from build123d import *

# Parameters (mm, degrees)
ESQUISSE1_R        = 0.825
ESQUISSE1_R_2      = 0.75
ESQUISSE1_W        = 38.13
ESQUISSE1_H        = 18.5
ESQUISSE1_W_2      = 17
ESQUISSE1_H_2      = 9
ESQUISSE1_W_3      = 2
ESQUISSE1_H_3      = 5
BOSS_EXTRU_1_DEPTH = 2
CHANFREIN1_SIZE    = 2
ESQUISSE2_R        = 1.65
BOSS_EXTRU_2_DEPTH = 2
CONG_1_R           = 2
CONG_4_R           = 2


with BuildPart() as part:
    # Esquisse1 → Boss.-Extru.1 (new body)
    # profile 1 of 3: a face of its own
    with BuildSketch(Plane(origin=(0, 0, 0), x_dir=(1, 0, 0), z_dir=(0, 1, 0))):
        Polygon((-11.996169772, 14.323981369), (31.213830228, 14.323981369), (35.738830228, 9.823981369), (83.213830228, 9.823981369), (83.213830228, -3.176018631), (35.738830228, -3.176018631), (31.213830228, -7.676018631), (-11.996169772, -7.676018631), align=None)
        with Locations(Location((-10.726169772, 11.303981369, 0), (0, 0, 270))):
            Circle(ESQUISSE1_R, mode=Mode.SUBTRACT)
        with Locations(Location((29.943830228, 11.303981369, 0), (0, 0, 270))):
            Circle(ESQUISSE1_R, mode=Mode.SUBTRACT)
        with Locations(Location((29.943830228, -4.656018631, 0), (0, 0, 270))):
            Circle(ESQUISSE1_R, mode=Mode.SUBTRACT)
        with Locations(Location((-10.726169772, -4.656018631, 0), (0, 0, 270))):
            Circle(ESQUISSE1_R, mode=Mode.SUBTRACT)
        with Locations(Location((33.943830228, 3.323981369, 0), (0, 0, 270))):
            Circle(ESQUISSE1_R_2, mode=Mode.SUBTRACT)
        with Locations(Location((54.533830228, 3.323981369, 0), (0, 0, 270))):
            Circle(ESQUISSE1_R_2, mode=Mode.SUBTRACT)
        with Locations(Location((60.533830228, 3.323981369, 0), (0, 0, 270))):
            Circle(ESQUISSE1_R_2, mode=Mode.SUBTRACT)
        with Locations(Location((81.123830228, 3.323981369, 0), (0, 0, 270))):
            Circle(ESQUISSE1_R_2, mode=Mode.SUBTRACT)
        with Locations((9.608830228, 3.323981369)):
            Rectangle(ESQUISSE1_W, ESQUISSE1_H, mode=Mode.SUBTRACT)
        with Locations((44.238830228, 3.323981369)):
            Rectangle(ESQUISSE1_W_2, ESQUISSE1_H_2, mode=Mode.SUBTRACT)
        with Locations((70.828830228, 3.323981369)):
            Rectangle(ESQUISSE1_W_2, ESQUISSE1_H_2, mode=Mode.SUBTRACT)
    # profile 2 of 3: a face of its own
    with BuildSketch(Plane(origin=(0, 0, 0), x_dir=(1, 0, 0), z_dir=(0, 1, 0))):
        with Locations((-12.996169772, 3.323981369)):
            Rectangle(ESQUISSE1_W_3, ESQUISSE1_H_3)
    # profile 3 of 3: a face of its own
    with BuildSketch(Plane(origin=(0, 0, 0), x_dir=(1, 0, 0), z_dir=(0, 1, 0))):
        with Locations((84.213830228, 3.323981369)):
            Rectangle(ESQUISSE1_W_3, ESQUISSE1_H_3)
    extrude(amount=BOSS_EXTRU_1_DEPTH)

    # Chanfrein1
    chanfrein1_edges = [part.edges().sort_by_distance(p)[0] for p in [
        (83.213830228, 1, -9.823981369),
        (83.213830228, 1, 3.176018631),
    ]]
    chamfer(chanfrein1_edges, length=CHANFREIN1_SIZE)

    # Esquisse2 → Boss.-Extru.2 (add)
    with BuildSketch(Plane(origin=(85.213830228, 0, 0), x_dir=(0, 0, -1), z_dir=(1, 0, 0))):
        Polygon((5.823981369, 0), (0.823981369, 0), (2.323981369, -2), (2.323981369, -9), (0.823981369, -9), (0.823981369, -14), (5.823981369, -14), (5.823981369, -9), (4.323981369, -9), (4.323981369, -2), align=None)
        with Locations((3.323981369, -11.5)):
            Circle(ESQUISSE2_R, mode=Mode.SUBTRACT)
    boss_extru_2 = extrude(amount=-BOSS_EXTRU_2_DEPTH)

    # Symétrie1: Boss.-Extru.2 across plane
    add(boss_extru_2.mirror(Plane(origin=(35.738830228, 2, 0), x_dir=(0, 0, 1), z_dir=(-1, 0, 0))))

    # Congé1
    # the kernel refuses this fillet: 2 mm, written as the material it takes off along each edge
    with BuildSketch(Plane(origin=(90.213830228, -14, -5.823981369), x_dir=(0, 0, 1), z_dir=(-1, 0, 0)), Plane(origin=(90.213830228, -14, -0.823981369), x_dir=(0, 1, 0), z_dir=(-1, 0, 0))) as cong_1_piece_1:
        with BuildLine():
            CenterArc((CONG_1_R, CONG_1_R), CONG_1_R, 180, 90)
            Line((0, CONG_1_R), (-CONG_1_R * 0.02, CONG_1_R))
            Line((-CONG_1_R * 0.02, CONG_1_R), (-CONG_1_R * 0.02, -CONG_1_R * 0.02))
            Line((-CONG_1_R * 0.02, -CONG_1_R * 0.02), (CONG_1_R, -CONG_1_R * 0.02))
            Line((CONG_1_R, -CONG_1_R * 0.02), (CONG_1_R, 0))
        make_face()
    extrude(amount=12, mode=Mode.SUBTRACT)
    with BuildSketch(Plane(origin=(90.055059411, -9, -5.823981369), x_dir=(0, -1, 0), z_dir=(-1, 0, 0)), Plane(origin=(-18.577398955, -9, -0.823981369), x_dir=(0, -1, 0), z_dir=(1, 0, 0))) as cong_1_piece_2:
        with BuildLine():
            CenterArc((1.936491673, 2), CONG_1_R, 194.477512186, 75.522487814)
            Line((0, 1.5), (-0.038729833, 1.49))
            ThreePointArc((-0.038729833, 1.49), (-0.04, 0.75), (-0.04, 0))
            Line((-0.04, 0), (0, -0.04))
            Line((0, -0.04), (1.936491673, -0.04))
            Line((1.936491673, -0.04), (1.936491673, 0))
        make_face()
    extrude(amount=11.682458366, mode=Mode.SUBTRACT)
    with BuildSketch(Plane(origin=(90.055059411, -9, -0.823981369), x_dir=(0, -1, 0), z_dir=(-1, 0, 0)), Plane(origin=(-18.577398955, -9, -5.823981369), x_dir=(0, -1, 0), z_dir=(1, 0, 0))) as cong_1_piece_3:
        with BuildLine():
            CenterArc((1.936491673, -2), CONG_1_R, 90, 75.522487814)
            Line((0, -1.5), (-0.038729833, -1.49))
            ThreePointArc((-0.038729833, -1.49), (-0.04, -0.75), (-0.04, 0))
            Line((-0.04, 0), (0, 0.04))
            Line((0, 0.04), (1.936491673, 0.04))
            Line((1.936491673, 0.04), (1.936491673, 0))
        make_face()
    extrude(amount=11.682458366, mode=Mode.SUBTRACT)
    with BuildSketch(Plane(origin=(-18.736169772, -14, -5.823981369), x_dir=(0, 0, 1), z_dir=(1, 0, 0)), Plane(origin=(-18.736169772, -14, -0.823981369), x_dir=(0, 1, 0), z_dir=(1, 0, 0))) as cong_1_piece_4:
        with BuildLine():
            CenterArc((CONG_1_R, -CONG_1_R), CONG_1_R, 90, 90)
            Line((0, -CONG_1_R), (-CONG_1_R * 0.02, -CONG_1_R))
            Line((-CONG_1_R * 0.02, -CONG_1_R), (-CONG_1_R * 0.02, CONG_1_R * 0.02))
            Line((-CONG_1_R * 0.02, CONG_1_R * 0.02), (CONG_1_R, CONG_1_R * 0.02))
            Line((CONG_1_R, CONG_1_R * 0.02), (CONG_1_R, 0))
        make_face()
    extrude(amount=12, mode=Mode.SUBTRACT)

    # Congé4
    cong_4_edges = [part.edges().sort_by_distance(p)[0] for p in [
        (84.213830228, -9, -4.323981369),
        (84.213830228, -9, -2.323981369),
        (-12.736169772, -9, -4.323981369),
        (-12.736169772, -9, -2.323981369),
    ]]
    fillet(cong_4_edges, radius=CONG_4_R)


solid = part.part
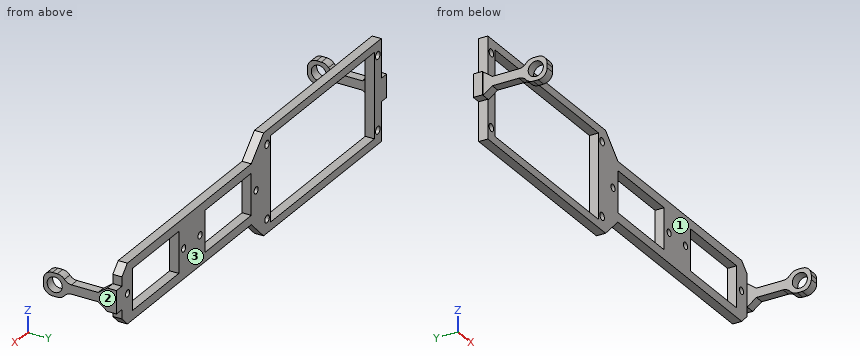
Can you work these out from the model? Positions are in its coordinate system, mm. Face numbers are marked on the shaded views. Give positions to 0.01 mm unless a question says otherwise; leave off trailing zeros. Order: outer loops, then holes, each group sorted by start corner. A loop starts at its lowest first (then second) coordinate and runs counter-clockwise, first axis right, second up. Notation, with made-up numbers: M 60.5,-33 L 99.5,-33 A15 cw 99.5,-23 Z; hole C 73,42.25 d3. An arc over 180 degrees is marked long. One line per item, written item: value.
Item 1: For pin 1 (2 mm diameter, centred on y = -11.5, z = -3.32, fed in from -X); pin 2 (6 mm diameter, centred on x = 46, y = -0.5, fed in from -Z); pin 3 (2 mm diameter, centred on y = 0.5, z = 4, fed in from -X), each with a flat end and sliding along its axis, tell me the tip position at first contact or that it passes through.
Verdict:
pin 1: through
pin 2: z = -9.82
pin 3: x = -12
Item 2: Please list where these lines run through material, in increasing order: line 1 (Z direction, x = 14, y = 1.25); line 2 (X direction, y = -3, z = -2.75); line 3 (Y direction, x = 60.5, z = 2).
Verdict:
line 1: -14.32 to -12.57, 5.93 to 7.68
line 2: -13.74 to -11.74, 83.21 to 85.21
line 3: 0 to 2
Item 3: If we section it at A-A on y = -6.5: Write out the boundary of the cut face in (x, z).
Verdict:
outline: M -13.74,-4.32 L -11.74,-4.32 L -11.74,-2.32 L -13.74,-2.32 Z; M 83.21,-4.32 L 85.21,-4.32 L 85.21,-2.32 L 83.21,-2.32 Z
Item 4: If we section it at B-B on x = 2: Write out the boundary of the cut face in (y, z).
Verdict:
outline: M 0,-14.32 L 2,-14.32 L 2,-12.57 L 0,-12.57 Z; M 0,5.93 L 2,5.93 L 2,7.68 L 0,7.68 Z
Item 5: If we mould it in two halves opening along X, with no side actions, what happens to the marked faces 1, 2 and 3? For each: pulls with the +X half, pulls with the -X half, needs draft (parallel to the pull), parting line crosses it, or undercut.
Verdict:
face 1: undercut
face 2: pulls with the +X half
face 3: needs draft
